Source: three-view drawing plus pictorial views. Frame: mm from the lowest corner of the part. Coordinates: 2 decimals unless noted, no trailing zeros. Order: outer loops, then holes, each group sorted by start corner. A loop starts at its lowest first (then second) coordinate and runs counter-clockwise, first axis right, second up. Notation, with made-up numbers: (82.25, 68) -> (127.25, 68) arc R28 ccw to (127.25, 86) -> close; hole circle Ø5 at (5, 54). An arc over 180 degrees is marked (long way). Use one line per item in the form item = value. Start each with the question number.
1) Section query B-B on x = 139.5. Output: boundary loops of the cut face in (y, z).
2) Pin query (flat end, axial travel): pin 1 (5 mm diameter, centred on x = 46, z = 33.5, fed in from -Y); pin 2 (3 mm diameter, centred on x = 4.5, z = 25.5, fed in from +Y); pin 3 (4 mm diameter, centred on y = 8.5, z = 48, fed in from -X). Return the tip coordinate at first contact, or that it passes through.
3) Section query A-A on z = 25.4. Output: boundary loops of the cut face in (x, y).
4) Ray query, line 1 along Z through (x, y) = (122.5, 7.75); line 2 along X through (y, z) = (10.75, 45); line 3 along X through (y, z) = (10.25, 22). Return the intervals inside material, ascending.
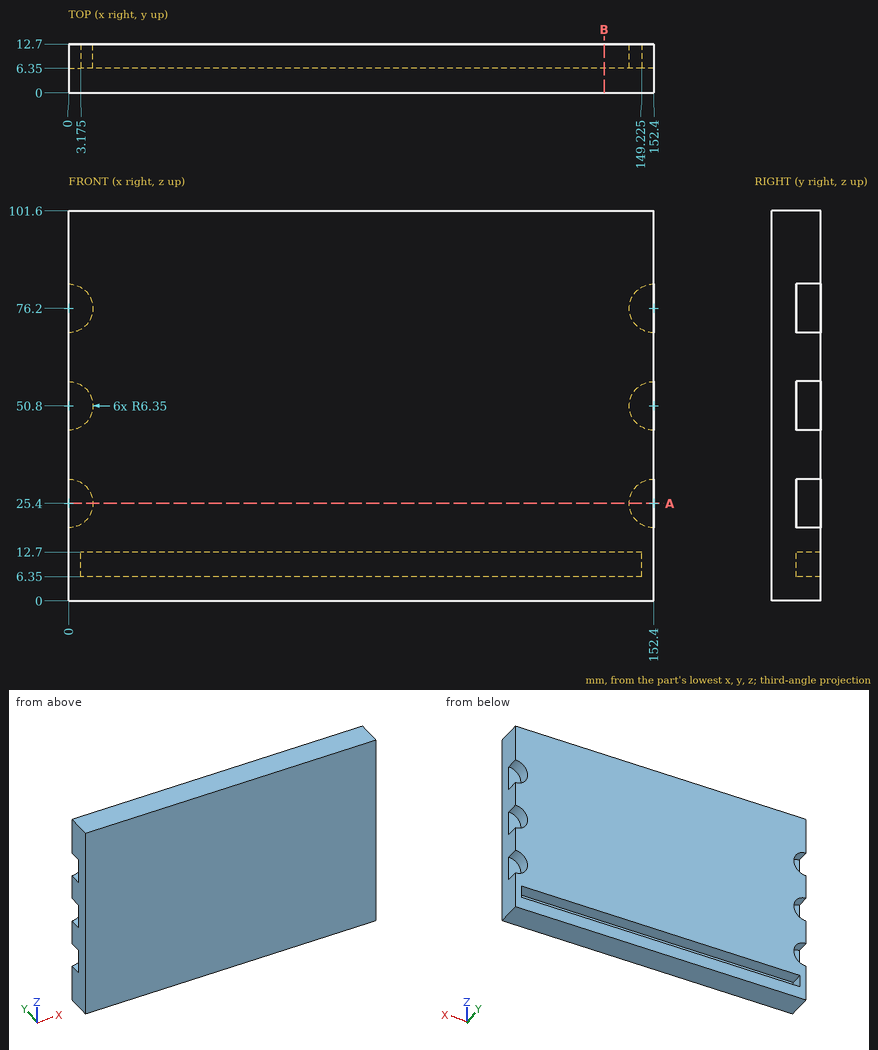
Answers below:
q1.outline = (0, 0) -> (12.7, 0) -> (12.7, 6.35) -> (6.35, 6.35) -> (6.35, 12.7) -> (12.7, 12.7) -> (12.7, 101.6) -> (0, 101.6) -> close
q2.pin_1 = 0
q2.pin_2 = 6.35
q2.pin_3 = 4.16
q3.outline = (0, 0) -> (152.4, 0) -> (152.4, 6.35) -> (146.05, 6.35) -> (146.05, 12.7) -> (6.35, 12.7) -> (6.35, 6.35) -> (0, 6.35) -> close
q4.line_1 = 0 to 6.35, 12.7 to 101.6
q4.line_2 = 2.59 to 149.81
q4.line_3 = 5.36 to 147.04
